```python
from build123d import *

# Parameters (mm, degrees)
F0_W     = 3.175
F0_H     = 2.978667
F0_W_2   = 10.16
F0_H_2   = 7.62
F0_H_3   = 3.175
F0_W_3   = 3.372148
F1_DEPTH = 12.7
F2_W     = 6.884132
F2_H     = 8.857906
F3_DEPTH = 25.4


with BuildPart() as f1:
    # F0 (on Top) → F1 (new body)
    with BuildSketch(Plane.XY):
        with Locations((-11.7475, 1.489333)):
            Rectangle(F0_W, F0_H)
        with Locations((-5.08, 1.489333)):
            Rectangle(F0_W_2, F0_H)
        with Locations((-11.7475, -3.81)):
            Rectangle(F0_W, F0_H_2)
        Polygon((2.891317, 2.978667), (0, 2.978667), (0, 0), (3.175, 0), align=None)
        with Locations((-11.7475, -9.2075)):
            Rectangle(F0_W, F0_H_3)
        with Locations((-8.473926, -9.2075)):
            Rectangle(F0_W_3, F0_H_3)
        Polygon((3.175, 0), (0, 0), (1.27, -13.335), (1.27, -10.16), (4.142619, -10.16), align=None)
        Polygon((14.394098, 2.978667), (2.891317, 2.978667), (3.175, 0), (14.394098, 0), align=None)
        Polygon((1.27, -10.16), (1.27, -13.335), (4.445, -13.335), (4.142619, -10.16), align=None)
        Polygon((4.445, -10.16), (4.142619, -10.16), (4.445, -13.335), align=None)
    extrude(amount=F1_DEPTH)

    # F2 (on Top) → F3 (cut)
    with BuildSketch(Plane.XY):
        with Locations((3.442066, -11.987058)):
            Rectangle(F2_W, F2_H)
    extrude(amount=F3_DEPTH, mode=Mode.SUBTRACT)


solid = f1.part
```
Part model, mm, in its own coordinate system. A direction names the side the tool comes from. Coordinates: 2 decimals unless noted, no trailing zeros. Order: outer loops, then holes, each group sorted by start corner. A loop starts at its lowest first (then second) coordinate and runs counter-clockwise, first axis right, second up. Notation, with made-up numbers: (-39, 31.5) - (-17, 31.5) arc R13 cw to (-17, 50.5) - close; hole circle Ø1 at (36.25, -28.5). An arc over 180 degrees is marked (long way). Return JSON: item names as keys, results as strings. Group by question number.
Item 1: Drill centre lines: probe 1 along Y at (x, z) = (-10, 5) (3 decimals); probe 2 along X at (y, z) = (-7.5, 2.5) (3 decimals); probe 3 along X at (y, z) = (-8.5, 9) (3 decimals). Where is each one in solid material? Low to high. Write a range as from..to.
Item 2: Cut at D-D (y = -9.25). List the corners of the cut face in (x, z) (3 decimals), plus the area to 3 significant figures.
Item 3: Which spindle directions (+Z, -Z, +X, -X, +Y, -Y) get a long thin tool onto all of the face, cutting with end or side? Do faces 4 (the face through (-10.16, -4, 6)), 5 (the face through (2, -7.558, 6)), 6 (the face through (-8, -7.62, 6)). Say none if no direction does.
Item 4: Pin check, flat tips, straight feed: pin 1 (5.5 mm diameter, centred on x = 6, z = 9.5, fed in from -Y); pin 2 (4 mm diameter, centred on y = -5, z = 8.5, fed in from +X); pin 3 (2.5 mm diameter, centred on y = -9.5, z = 9.5, fed in from +X). Stop position of each tip, or through.
Item 5: Cut at B-B (y = -4). List the corners of the cut face in (x, z) (3 decimals).
Item 6: Pull direction X, two halves, no side cores. Call faces 1 (the face through (0.355, -3.726, 6.261)), 2 (the face through (14.394, 1, 6)), 3 (the face through (9, 0, 6)): pulls with the +X half, pulls with the -X half, needs draft (parallel to the pull), parting line crosses it, or undercut.
Item 7: Cut at C-C (x = -0.75). List the corners of the cut face in (y, z).
Item 8: Cut at A-A (z = 5.75). List the corners of the cut face in (x, y) (3 decimals).
Check values:
{
 "1": {"probe 1": "y = -10.795..-7.62, 0..2.979", "probe 2": "x = -13.335..-10.16, 0.714..3.889", "probe 3": "x = -13.335..-6.788"},
 "2": {"outline": "(-13.335, 0) - (-6.788, 0) - (-6.788, 12.7) - (-13.335, 12.7) - close", "area": "83.1 mm2"},
 "3": {"face 4": "+Z, -Z", "face 5": "+Z, -Z, +X, -Y", "face 6": "+Z, -Z, +X"},
 "4": {"pin 1": "stops at y = -7.56", "pin 2": "stops at x = 3.84", "pin 3": "stops at x = -6.79"},
 "5": {"outline": "(-13.335, 0) - (-10.16, 0) - (-10.16, 12.7) - (-13.335, 12.7) - close; (0.381, 0) - (3.556, 0) - (3.556, 12.7) - (0.381, 12.7) - close"},
 "6": {"face 1": "undercut", "face 2": "pulls with the +X half", "face 3": "needs draft"},
 "7": {"outline": "(0, 0) - (2.98, 0) - (2.98, 12.7) - (0, 12.7) - close"},
 "8": {"outline": "(-13.335, -10.795) - (-6.788, -10.795) - (-6.788, -7.62) - (-10.16, -7.62) - (-10.16, 0) - (0, 0) - (0.72, -7.558) - (3.895, -7.558) - (3.175, 0) - (14.394, 0) - (14.394, 2.979) - (-13.335, 2.979) - close"}
}
